Here's the drawing with two shaded views (mm, measured from the low corner). I have some questions. A direction names the side the tool comes from. Give positions to 0.01 mm unless a question says otherwise; leave off trailing zeros. Write each loop counter-clockwise with the first axis right and the second up, starting at its lowest first coordinate (ties: lowest second). Pieces come first, ordered by that corner, then holes. Notation, with made-up numbers: (88.25, 71) - (107.25, 71) arc R29 cw to (107.25, 107) - close; hole circle Ø1 at (85, 53). An arc over 180 degrees is marked (long way). Answer as a JSON object with one key per item and string values. Group by question number.
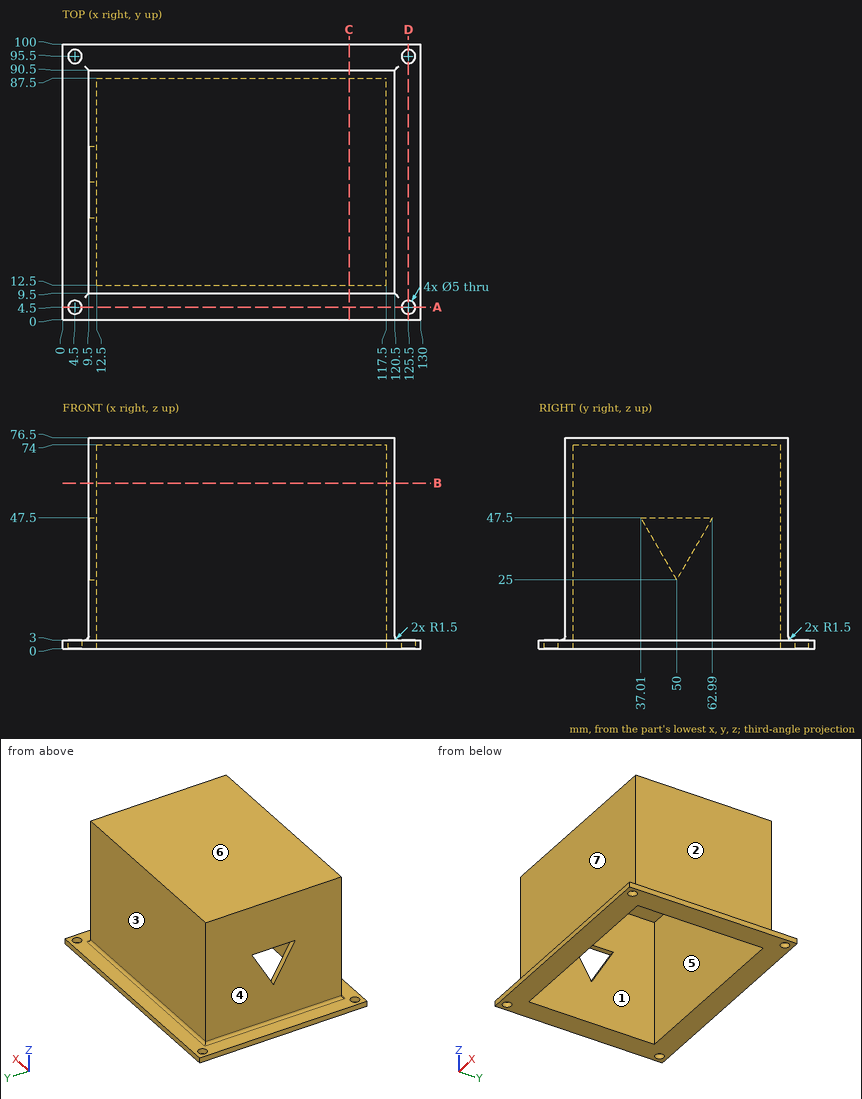
(1) I want a section at D-D, the plane x = 125.5. Please give me the cut outline in (y, z).
(2) I want a section at C-C, the plane x = 104. Please give me the cut outline in (y, z).
(3) I need wall thicknesses on L1, parallel to Y at x = 125.5, z = 1.2; L2, parallel to Y at x = 100.5, z = 11; L3, parallel to X at y = 44, z = 58. Which ranges of each line are inside material? Lowest first, please.
(4) I want a section at B-B, the plane z = 60. Please give me the cut outline in (x, y).
(5) I want a section at A-A, the plane y = 4.5. Please give me the cut outline in (x, z).
(6) For the marked faces 1, 2, 3 and 4, which set-ups out of +Z, -Z, +X, -X, +Y, -Y let a thin tool reach every point of the face, with its end or its side?
(7) Will these pins go through, and if not, where does the flat tip stop? P1, Ø2, axis at y = 65.5, z = 58.5, coming from the +X side; P2, Ø6, axis at x = 89, z = 48.5, coming from the -Y side; P3, Ø1.5, axis at y = 85, z = 26, coming from the -X side; P4, Ø2.5, axis at x = 11, y = 53.5, coming from the -Z side.
(8) If we mould it in two halves opening along Y, with no side actions, what happens to the marked faces 5, 6 and 7? For each: +Y half, -Y half, draft (parallel to the pull), parting line (faces both ways), or undercut.
Entries:
{
 "1": {"outline": "(0, 0) - (2, 0) - (2, 3) - (0, 3) - close; (7, 0) - (93, 0) - (93, 3) - (7, 3) - close; (98, 0) - (100, 0) - (100, 3) - (98, 3) - close"},
 "2": {"outline": "(0, 0) - (12.5, 0) - (12.5, 74) - (87.5, 74) - (87.5, 0) - (100, 0) - (100, 3) - (92, 3) arc R1.5 cw to (90.5, 4.5) - (90.5, 76.5) - (9.5, 76.5) - (9.5, 4.5) arc R1.5 cw to (8, 3) - (0, 3) - close"},
 "3": {"L1": "0 to 2, 7 to 93, 98 to 100", "L2": "9.5 to 12.5, 87.5 to 90.5", "L3": "9.5 to 12.5, 117.5 to 120.5"},
 "4": {"outline": "(9.5, 9.5) - (120.5, 9.5) - (120.5, 90.5) - (9.5, 90.5) - close; hole (12.5, 12.5) - (117.5, 12.5) - (117.5, 87.5) - (12.5, 87.5) - close"},
 "5": {"outline": "(0, 0) - (2, 0) - (2, 3) - (0, 3) - close; (7, 0) - (123, 0) - (123, 3) - (7, 3) - close; (128, 0) - (130, 0) - (130, 3) - (128, 3) - close"},
 "6": {"face 1": "-Z", "face 2": "+Z, +X, +Y, -Y", "face 3": "+Z, +X, -X, +Y", "face 4": "+Z, -X, +Y, -Y"},
 "7": {"P1": "x = 120.5", "P2": "y = 9.5", "P3": "x = 9.5", "P4": "z = 0"},
 "8": {"face 5": "undercut", "face 6": "draft", "face 7": "-Y half"}
}
